```python
from build123d import *

# Parameters (mm, degrees)
ESBO_O1_R                = 12.5
ESBO_O1_R_2              = 0.9
ESBO_O1_R_3              = 0.25
RESSALTO_EXTRUS_O1_DEPTH = 50.6
ESBO_O2_R                = 3.5
RESSALTO_EXTRUS_O2_DEPTH = 2
ESBO_O3_R                = 2
RESSALTO_EXTRUS_O3_DEPTH = 11.8
ESBO_O4_R                = 4.25
RESSALTO_EXTRUS_O4_DEPTH = 2.8
CORTE_EXTRUS_O1_START    = -29.8
ESBO_O6_R                = 12.5
ESBO_O6_R_2              = 12.1
CORTE_EXTRUS_O1_DEPTH    = 29.8


with BuildPart() as part:
    # Esboço1 → Ressalto-extrusão1 (new body)
    with BuildSketch(Plane.XY):
        Circle(ESBO_O1_R)
        with Locations((0, 8.5)):
            Circle(ESBO_O1_R_2, mode=Mode.SUBTRACT)
        with Locations((0, -8.5)):
            Circle(ESBO_O1_R_2, mode=Mode.SUBTRACT)
        with Locations((8.5, 0)):
            Circle(ESBO_O1_R_3, mode=Mode.SUBTRACT)
        with Locations((-8.5, 0)):
            Circle(ESBO_O1_R_3, mode=Mode.SUBTRACT)
    extrude(amount=RESSALTO_EXTRUS_O1_DEPTH)

    # Esboço2 → Ressalto-extrusão2 (add)
    with BuildSketch(Plane.XY):
        Circle(ESBO_O2_R)
    extrude(amount=-RESSALTO_EXTRUS_O2_DEPTH)

    # Esboço3 → Ressalto-extrusão3 (add)
    with BuildSketch(Plane.XY):
        Circle(ESBO_O3_R)
    extrude(amount=-RESSALTO_EXTRUS_O3_DEPTH)

    # Esboço4 → Ressalto-extrusão4 (add)
    with BuildSketch(Plane.XY.offset(50.6)):
        Circle(ESBO_O4_R)
    extrude(amount=RESSALTO_EXTRUS_O4_DEPTH)

    # Esboço6 → Corte-extrusão1 (cut)
    with BuildSketch(Plane.XY.offset(50.6).offset(CORTE_EXTRUS_O1_START)):
        Circle(ESBO_O6_R)
        Circle(ESBO_O6_R_2, mode=Mode.SUBTRACT)
    extrude(amount=CORTE_EXTRUS_O1_DEPTH, mode=Mode.SUBTRACT)


solid = part.part
```
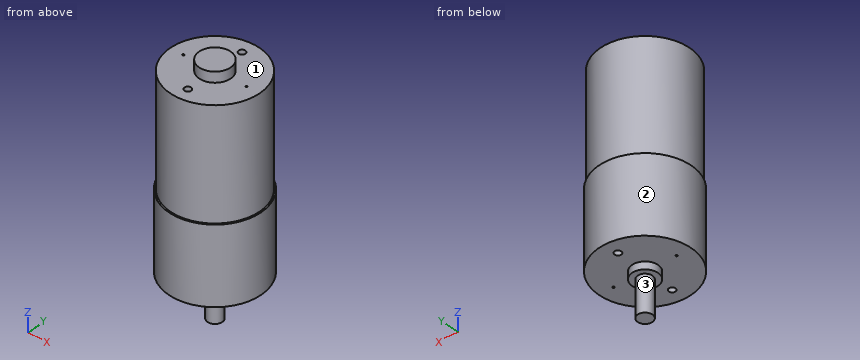
Check sheet for the modelled part. Datum: model origin and axes. Units: mm. Face numbers are marked on the shaded views. A direction names the side the tool comes from. Give positions to 0.01 mm unless a question says otherwise; leave off trailing zeros. Write each loop counter-clockwise with the first axis right and the second up, starting at its lowest first coordinate (ties: lowest second). Pieces come first, ordered by that corner, then holes. Notation, with made-up numbers: (-11.5, -25.5) - (34.5, -25.5) arc R22 ccw to (34.5, 13.5) - close; hole circle Ø4 at (8.5, -26.5). An arc over 180 degrees is marked (long way). Answer as a JSON object with one key per item and string values. Group by question number.
1) Depth check by flat-ended pin: P1, Ø10, axis at x = 9.5, z = 27, coming from the +Y side; P2, Ø1.6, axis at x = 0, y = -8.5, coming from the -Z side; P3, Ø12, axis at x = 1, z = -3.5, coming from the -Y side; P4, Ø4, axis at y = -5, z = 0.5, coming from the +X side. Enter the tip coordinate at first touch or a pass-through.
2) Sectioned sample at A-A (y = -8.5). Record the cut outline in (x, z).
3) Sectioned sample at C-C (z = -5.5). Record the cut outline in (x, y), then the cut area to 3 significant figures.
4) Sectioned sample at B-B (z = 27.5). Record the cut outline in (x, y), then the cut area to 3 significant figures.
5) Thickness scan on probe 1 along Y at (x, z) = (-0.25, 18); probe 2 along Z at (x, y) = (-7, 8); probe 3 along Z at (x, y) = (-0.5, 3.5). Record the ranges inside material, lowest first. Write a range as from..to.
6) Access from +Z, -Z, +X, -X, +Y, -Y to the whole of each face (thin tool, end or side, straight path). Record for the marked faces 1, 2 and 3.
7) Sectioned sample at D-D (z = 15.5). Record the cut outline in (x, y), then the cut area to 3 significant figures.
Geometry results:
{
 "1": {"P1": "stops at y = 11.23", "P2": "passes through", "P3": "stops at y = -12.5", "P4": "stops at x = 12.13"},
 "2": {"outline": "(-9.17, 0) - (-0.9, 0) - (-0.9, 50.6) - (-8.61, 50.6) - (-8.61, 20.8) - (-9.17, 20.8) - close; (0.9, 0) - (9.17, 0) - (9.17, 20.8) - (8.61, 20.8) - (8.61, 50.6) - (0.9, 50.6) - close"},
 "3": {"outline": "circle Ø4 at (0, 0)", "area": "12.6 mm^2"},
 "4": {"outline": "circle Ø24.2 at (0, 0); hole circle Ø0.5 at (-8.5, 0); hole circle Ø1.8 at (0, -8.5); hole circle Ø1.8 at (0, 8.5); hole circle Ø0.5 at (8.5, 0)", "area": "454 mm^2"},
 "5": {"probe 1": "y = -12.5..-9.36, -7.64..7.64, 9.36..12.5", "probe 2": "z = 0..50.6", "probe 3": "z = 0..53.4"},
 "6": {"face 1": "+Z", "face 2": "+Z, -Z", "face 3": "-Z"},
 "7": {"outline": "circle Ø25 at (0, 0); hole circle Ø0.5 at (-8.5, 0); hole circle Ø1.8 at (0, -8.5); hole circle Ø1.8 at (0, 8.5); hole circle Ø0.5 at (8.5, 0)", "area": "485 mm^2"}
}
